```python
from build123d import *

# Parameters (mm, degrees)
F0_W     = 80
F0_H     = 48
F0_R     = 2.5
F0_R_2   = 20
F1_DEPTH = 30
F2_DEPTH = 10
F3_SIZE  = 0.5
F4_R     = 4
F5_DEPTH = 10
F6_SIZE  = 0.5


with BuildPart() as f1:
    # F0 (on Right) → F1 (new body)
    with BuildSketch(Plane.YZ):
        Rectangle(F0_W, F0_H)
        with Locations((-21.650635, -12.5)):
            Circle(F0_R, mode=Mode.SUBTRACT)
        with Locations((21.650635, -12.5)):
            Circle(F0_R, mode=Mode.SUBTRACT)
        with Locations((-21.650635, 12.5)):
            Circle(F0_R, mode=Mode.SUBTRACT)
        Circle(F0_R_2, mode=Mode.SUBTRACT)
        with Locations((21.650635, 12.5)):
            Circle(F0_R, mode=Mode.SUBTRACT)
        with Locations((-21.650635, 12.5)):
            Circle(F0_R)
        with Locations((-21.650635, -12.5)):
            Circle(F0_R)
        with Locations((21.650635, 12.5)):
            Circle(F0_R)
        with Locations((21.650635, -12.5)):
            Circle(F0_R)
    extrude(amount=-F1_DEPTH)

    # F0 (on Right) → F2 (cut)
    with BuildSketch(Plane.YZ):
        with Locations((-21.650635, 12.5)):
            Circle(F0_R)
        with Locations((21.650635, 12.5)):
            Circle(F0_R)
        with Locations((21.650635, -12.5)):
            Circle(F0_R)
        with Locations((-21.650635, -12.5)):
            Circle(F0_R)
    extrude(amount=-F2_DEPTH, mode=Mode.SUBTRACT)

    # F3
    f3_edges = [f1.edges().sort_by_distance(p)[0] for p in [
        (-15, 20, 0),
        (0, -20, 0),
        (-30, -20, 0),
        (-5, -19.150635, 12.5),
        (0, -24.150635, 12.5),
        (-10, -24.150635, 12.5),
        (-5, -19.150635, -12.5),
        (0, -24.150635, -12.5),
        (-10, -24.150635, -12.5),
        (-5, 24.150635, 12.5),
        (0, 19.150635, 12.5),
        (-10, 19.150635, 12.5),
        (-5, 24.150635, -12.5),
        (0, 19.150635, -12.5),
        (-10, 19.150635, -12.5),
    ]]
    chamfer(f3_edges, length=F3_SIZE)

    # F4 (on face) → F5 (cut)
    with BuildSketch(Plane.XY.offset(24)):
        with Locations((-15, 30)):
            Circle(F4_R)
        with Locations((-15, -30)):
            Circle(F4_R)
    extrude(amount=-F5_DEPTH, mode=Mode.SUBTRACT)

    # F6
    f6_edges = [f1.edges().sort_by_distance(p)[0] for p in [
        (-11, 30, 19),
        (-19, 30, 24),
        (-19, 30, 14),
        (-11, -30, 19),
        (-19, -30, 24),
        (-19, -30, 14),
    ]]
    chamfer(f6_edges, length=F6_SIZE)


solid = f1.part
```
Geometry: final body of the model. Coordinates: model frame, mm. A direction names the side the tool comes from. Coordinates: 2 decimals unless noted, no trailing zeros. Order: outer loops, then holes, each group sorted by start corner. A loop starts at its lowest first (then second) coordinate and runs counter-clockwise, first axis right, second up.
Item 1: Material intervals for line 1 along Y through (x, z) = (-15, 17.75); line 2 along Y through (x, z) = (-9.25, -11); line 3 along Z through (x, y) = (-12.25, -7) (3 decimals), sorted ascending.
Answer:
line 1: y = -40 to -34, -26 to -9.22, 9.22 to 26, 34 to 40
line 2: y = -40 to -23.65, -19.65 to -16.7, 16.7 to 19.65, 23.65 to 40
line 3: z = -24 to -18.735, 18.735 to 24
Item 2: Contact query for flat-ended pins moving along their axis: P1, Ø1.2, axis at y = 22.5, z = -13, coming from the +X side; P2, Ø5, axis at x = -15, y = 30, coming from the +Z side. Output: stop coordinate, or through.
Answer:
P1: stops at x = -10
P2: stops at z = 14
Item 3: Section query A-A (y = 0). Output: boundary loops of the cut face in (x, z), then the cut area to 4 significant figures.
Answer:
outline: (-30, -24) - (0, -24) - (0, -20.5) - (-0.5, -20) - (-29.5, -20) - (-30, -20.5) - close; (-30, 20.5) - (-29.5, 20) - (-0.5, 20) - (0, 20.5) - (0, 24) - (-30, 24) - close
area: 239.5 mm2
Item 4: Section query D-D (x = -7). Output: boundary loops of the cut face in (y, z), then the cut area to 3 significant figures.
Answer:
outline: (-40, -24) - (40, -24) - (40, 24) - (-40, 24) - close; hole circle Ø5 at (-21.65, -12.5); hole circle Ø5 at (-21.65, 12.5); hole circle Ø40 at (0, 0); hole circle Ø5 at (21.65, -12.5); hole circle Ø5 at (21.65, 12.5)
area: 2,500 mm2
Item 5: Access query for faces 1 (the face through (-15, 40, 0)), 2 (the face through (-15, -30, 14)), 3 (the face through (-4.94, -20.5, 10.28)). Directions: +Z, -Z, +X, -X, +Y, -Y. A direction counts if a zero-diameter tool reaches every point of the face in a straight line with its end or side. Return the directions, or none.
Answer:
face 1: +Z, -Z, +X, -X, +Y
face 2: +Z
face 3: +X
Item 6: Section query B-B (x = -15). Output: boundary loops of the cut face in (y, z).
Answer:
outline: (-40, -24) - (40, -24) - (40, 24) - (34.5, 24) - (34, 23.5) - (34, 14.5) - (33.5, 14) - (26.5, 14) - (26, 14.5) - (26, 23.5) - (25.5, 24) - (-25.5, 24) - (-26, 23.5) - (-26, 14.5) - (-26.5, 14) - (-33.5, 14) - (-34, 14.5) - (-34, 23.5) - (-34.5, 24) - (-40, 24) - close; hole circle Ø40 at (0, 0)
Item 7: Section query C-C (z = 0). Output: boundary loops of the cut face in (x, y).
Answer:
outline: (-30, -40) - (0, -40) - (0, -20.5) - (-0.5, -20) - (-29.5, -20) - (-30, -20.5) - close; (-30, 20.5) - (-29.5, 20) - (-0.5, 20) - (0, 20.5) - (0, 40) - (-30, 40) - close
Item 8: Draft query along Z for faces 4 (the face through (-15, -40, 0)), 5 (the face through (-10, 22, 13)), 6 (the face through (-14.797, -4.336, -19.524)), 7 (the face through (-15, -1, 24)). Return one class per face: released by +Z, released by -Z, zero draft, split by the parting line, or undercut.
Answer:
face 4: zero draft
face 5: undercut
face 6: undercut
face 7: released by +Z
